Can you work these out from the model? Positions are in its coordinate system, mm. A direction names the side the tool comes from. Round coordinates to 2 decimals unless told otherwise and drop trailing zeros. Loops run counter-clockwise (first coordinate to the right, second up) from the corner with the lowest first, then second, coordinate; pieces in that order, holes last.
(1) I want a section at B-B on y = 20. Write out the boundary of the cut face in (x, z).
(2) I want a section at A-A on y = 0. Write out the boundary of the cut face in (x, z), plus the area to 3 significant figures.
(3) Thinking about a two-plate mould opening in Y: for faces 4 (the face through (24.24, -37.55, 2.54)), 5 (the face through (-43, -1, 5)), 6 (the face through (10, -25, 0)), 7 (the face through (-25.25, 42.92, 3.82)), which applies, released by +Y, released by -Y, zero draft, split by the parting line, or undercut?
(4) Will these pins go through, and if not, where does the flat tip stop? pin 1 Ø3 at (x, y) = (-44, -1) entering from +Z; pin 2 Ø4 at (y, z) = (0, 7.5) entering from +X; pin 3 Ø1.5 at (x, z) = (28, 8) entering from -Y.
(5) If I drill on line 1 along Y through (x, z) = (0, 1.55); line 2 along Y through (x, z) = (0, 7.75); line 3 along X through (y, z) = (26.5, 1.5), over which ranges is the centre line in solid material (lowest first)?
(6) I want a section at C-C on z = 7.5. Write out the boundary of the cut face in (x, y).
(7) Which directions (+Z, -Z, +X, -X, +Y, -Y) give clear straight access to the entire face, cutting with the end or side of a thin tool? Please do faces 1 (the face through (-41.306, -24.599, 5.07)), 2 (the face through (-39.3, -0.2, 7.5)), 3 (the face through (-23.846, 7.509, 2.465)).
(8) I want a section at D-D on y = -51. Write out the boundary of the cut face in (x, z), plus the area to 3 significant figures.
Autodesk Inventor part; units mm, degrees
ref_plane "YZ Plane" through (0, 0, 0) normal (1, 0, 0) x (0, 1, 0)
ref_plane "XZ Plane" through (0, 0, 0) normal (0, 1, 0) x (-1, 0, 0)
ref_plane "XY Plane" through (0, 0, 0) normal (0, 0, 1) x (1, 0, 0)
sketch "Sketch1" plane through (0, 0, 0) normal (0, 0, 1) x (1, 0, 0)
  circle A0 centre (0, 0) radius 12.5
  circle A1 centre (-30, 0) radius 3
  circle A2 centre (-15, -25.9808) radius 3
  circle A3 centre (15, -25.9808) radius 3
  circle A4 centre (30, 0) radius 3
  circle A5 centre (15, 25.9808) radius 3
  circle A6 centre (-15, 25.9808) radius 3
  line L0 (0, 57.5) -> (49.7965, 28.75)
  line L1 (49.7965, 28.75) -> (49.7965, -28.75)
  line L2 (49.7965, -28.75) -> (0, -57.5)
  line L3 (0, -57.5) -> (-49.7965, -28.75)
  line L4 (-49.7965, -28.75) -> (-49.7965, 28.75)
  line L5 (-49.7965, 28.75) -> (0, 57.5)
  point P0 (49.7965, 0)
  dimension "d0" = 25
  dimension "d2" = 6
  dimension "d6" = 360
  dimension "d15" = 30
  dimension "d33" = 115
extrude "Extrusion1" add sketch "Sketch1" along normal blind 10 contours A1 | A2 | A3 | A4 | A5 | A6 | L0 L1 L2 L3 L4 L5
sketch "Sketch7" plane through (0, 0, 10) normal (0, 0, 1) x (1, 0, 0)
  circle A0 centre (0, 51) radius 3
  circle A1 centre (-44.1673, 25.5) radius 3
  circle A2 centre (-44.1673, -25.5) radius 3
  circle A3 centre (0, -51) radius 3
  circle A4 centre (44.1673, -25.5) radius 3
  circle A5 centre (44.1673, 25.5) radius 3
  line L0 (0, 51) -> (0, -51)
  point P0 (0, 0)
  dimension "d42" = 6
  dimension "d46" = 360
  dimension "d96" = 102
extrude "Extrusion6" cut sketch "Sketch7" against normal through all
sketch "Sketch9" plane through (0, 0, 0) normal (0, 0, -1) x (-1, 0, 0)
  circle A0 centre (0, 0) radius 25
  dimension "d56" = 50
extrude "Extrusion8" cut sketch "Sketch9" against normal blind 5
sketch "Sketch14" plane through (0, 0, 10) normal (0, 0, 1) x (1, 0, 0)
  circle A0 centre (-45.7965, 0) radius 2.5
  circle A1 centre (-22.8982, -39.6609) radius 2.5
  circle A2 centre (22.8982, -39.6609) radius 2.5
  circle A3 centre (45.7965, 0) radius 2.5
  circle A4 centre (22.8982, 39.6609) radius 2.5
  circle A5 centre (-22.8982, 39.6609) radius 2.5
  line L0 (-49.7965, 28.75) -> (-49.7965, -28.75)
  point P0 (0, 0)
  point P1 (-45.7965, 0)
  dimension "d81" = 5
  dimension "d85" = 360
  dimension "d97" = 4
extrude "Extrusion13" cut sketch "Sketch14" against normal through all
sketch "Sketch15" plane through (0, 0, 10) normal (0, 0, 1) x (1, 0, 0)
  circle A0 centre (-22.8982, 39.6609) radius 2.5
  circle A1 centre (-22.8982, 39.6609) radius 6.5
  circle A2 centre (-45.7965, 0) radius 6.5
  circle A3 centre (-22.8982, -39.6609) radius 6.5
  circle A4 centre (22.8982, -39.6609) radius 6.5
  circle A5 centre (45.7965, 0) radius 6.5
  circle A6 centre (22.8982, 39.6609) radius 6.5
  point P0 (0, 0)
  dimension "d89" = 13
  dimension "d92" = 360
extrude "Extrusion14" cut sketch "Sketch15" against normal blind 5 contours A0 | A1 | A2 | A3 | A4 | A5 | A6
properties part number "TA01" material "ABS Plastic"
Filled sheet:
1. outline: (-49.8, 0) - (-15, 0) - (-15, 5) - (15, 5) - (15, 0) - (49.8, 0) - (49.8, 10) - (-49.8, 10) - close
2. outline: (-49.8, 0) - (-48.3, 0) - (-48.3, 5) - (-49.8, 5) - close; (-43.3, 0) - (-25, 0) - (-25, 5) - (-12.5, 5) - (-12.5, 10) - (-39.3, 10) - (-39.3, 5) - (-43.3, 5) - close; (12.5, 5) - (25, 5) - (25, 0) - (43.3, 0) - (43.3, 5) - (39.3, 5) - (39.3, 10) - (12.5, 10) - close; (48.3, 0) - (49.8, 0) - (49.8, 5) - (48.3, 5) - close
2. area: 466 mm2
3. face 4: undercut
3. face 5: undercut
3. face 6: zero draft
3. face 7: released by +Y
4. pin 1: stops at z = 5
4. pin 2: stops at x = 39.61
4. pin 3: stops at y = -36.83
5. line 1: y = -57.5 to -54, -48 to -25, 25 to 48, 54 to 57.5
5. line 2: y = -57.5 to -54, -48 to -12.5, 12.5 to 48, 54 to 57.5
5. line 3: x = -49.8 to -47, -41.34 to 41.34, 47 to 49.8
6. outline: (-49.8, -28.75) - (-29.34, -40.56) arc R6.5 cw (long way) to (-20.46, -45.69) - (0, -57.5) - (20.46, -45.69) arc R6.5 cw (long way) to (29.34, -40.56) - (49.8, -28.75) - (49.8, -5.12) arc R6.5 cw (long way) to (49.8, 5.12) - (49.8, 28.75) - (29.34, 40.56) arc R6.5 cw (long way) to (20.46, 45.69) - (0, 57.5) - (-20.46, 45.69) arc R6.5 cw (long way) to (-29.34, 40.56) - (-49.8, 28.75) - (-49.8, 5.12) arc R6.5 cw (long way) to (-49.8, -5.12) - close; hole circle Ø6 at (-44.17, -25.5); hole circle Ø6 at (-44.17, 25.5); hole circle Ø25 at (0, 0); hole circle Ø6 at (0, -51); hole circle Ø6 at (0, 51); hole circle Ø6 at (44.17, -25.5); hole circle Ø6 at (44.17, 25.5)
7. face 1: +Z, -Z
7. face 2: +Z
7. face 3: -Z
8. outline: (-11.26, 0) - (-3, 0) - (-3, 10) - (-11.26, 10) - close; (3, 0) - (11.26, 0) - (11.26, 10) - (3, 10) - close
8. area: 165 mm2
